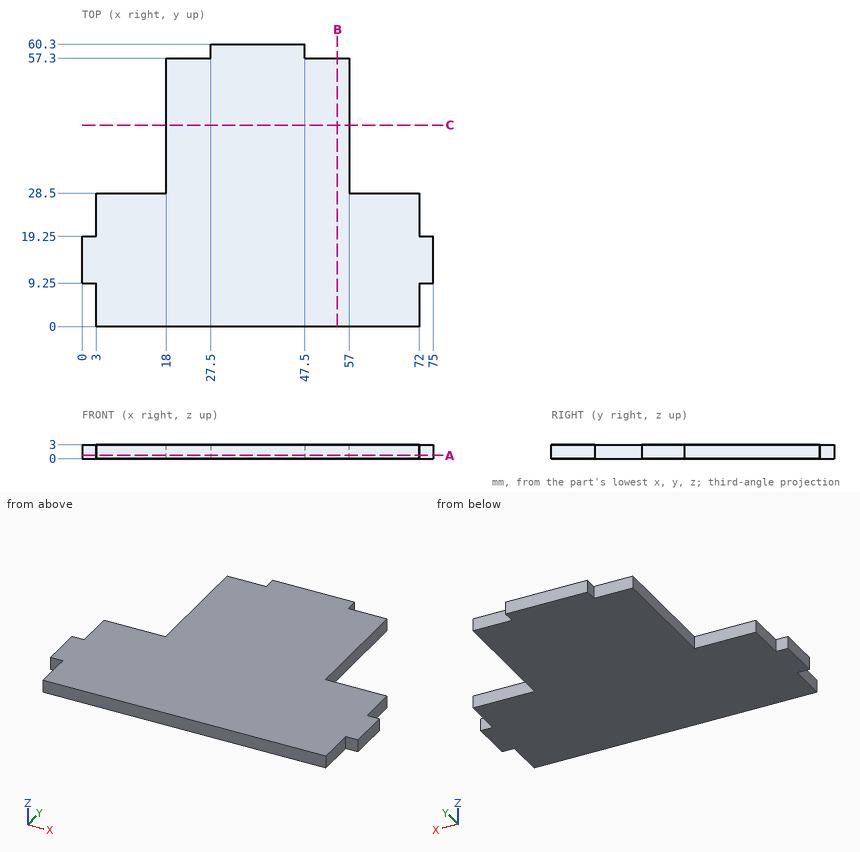
Can you work these out from the drawing? Everything is in mm from the part's minimum corner. Coordinates: 2 decimals unless noted, no trailing zeros. Write each loop counter-clockwise with the first axis right and the second up, starting at its lowest first coordinate (ties: lowest second). Pieces come first, ordered by that corner, then holes. Notation, with made-up numbers: (42.25, -28) -> (65.25, -28) arc R8 cw to (65.25, -13) -> close; hole circle Ø6 at (-40, 64). An arc over 180 degrees is marked (long way). Return JSON: item names as keys, results as strings.
(1) Imagine slicing it at B-B, the plane x = 54.5. Please give me the cut outline in (y, z).
Numbers:
{"outline": "(0, 0) -> (57.3, 0) -> (57.3, 3) -> (0, 3) -> close"}
(2) I need wall thicknesses on L1, parallel to X at y = 38.5, z = 2.75; L2, parallel to Y at x = 21, z = 0.75; L3, parallel to Y at x = 5.5, z = 2.85. Which ranges of each line are inside material? Lowest first, please.
Numbers:
{"L1": "x = 18 to 57", "L2": "y = 0 to 57.3", "L3": "y = 0 to 28.5"}
(3) Imagine slicing it at C-C, the plane y = 43. Please give me the cut outline in (x, z).
Numbers:
{"outline": "(18, 0) -> (57, 0) -> (57, 3) -> (18, 3) -> close"}
(4) I'm going to push flat-ended pins straight in: pin 1 (1.5 mm diameter, centred on y = 58.5, z = 2, fed in from +X); pin 2 (1.5 mm diameter, centred on x = 2, z = 1, fed in from +Y); pin 3 (1.5 mm diameter, centred on y = 59.5, z = 1.5, fed in from -X). Where does each tip first touch, or does it pass through?
Numbers:
{"pin 1": "stops at x = 47.5", "pin 2": "stops at y = 19.25", "pin 3": "stops at x = 27.5"}
(5) Imagine slicing it at A-A, the plane z = 0.7. Please give me the cut outline in (x, y), then the cut area to 3 significant figures.
Numbers:
{"outline": "(0, 9.25) -> (3, 9.25) -> (3, 0) -> (72, 0) -> (72, 9.25) -> (75, 9.25) -> (75, 19.25) -> (72, 19.25) -> (72, 28.5) -> (57, 28.5) -> (57, 57.3) -> (47.5, 57.3) -> (47.5, 60.3) -> (27.5, 60.3) -> (27.5, 57.3) -> (18, 57.3) -> (18, 28.5) -> (3, 28.5) -> (3, 19.25) -> (0, 19.25) -> close", "area": "3,210 mm2"}
